Input: dimensioned drawing with shaded views. Units: mm. Origin: part minimum x, y, z. Give positions to 0.01 mm unless a question says otherwise; leave off trailing zeros. Order: outer loops, then holes, each group sorted by start corner. A loop starts at its lowest first (then second) coordinate and runs counter-clockwise, first axis right, second up. Notation, with made-up numbers: M -9,8.5 L 9,8.5 A17 cw 9,12.5 Z; hole C 21.25,10 d11. An arc over 180 degrees is marked long. Answer in a Markdown table with one row per item. Add a question column.
(1) Material intervals for line 1 along Y through (x, z) = (6.5, 1.75); line 2 along Y through (x, z) = (7, 0.3) (1 decimal); line 3 along X through (y, z) = (21, 0.25) (1 decimal), sorted ascending.
(2) Mould query, pull axis Y, two halves, no side actions, for the marked faces 1, 2 and 3. Classes: pulls with the +Y half, pulls with the -Y half, needs draft (parallel to the pull), parting line crosses it, or undercut.
(3) Section query D-D, the plane y = 2.25. Return loops of the section in (x, z) (1 decimal), plus the area to 3 significant figures.
(4) Pin query (flat end, axial travel): P1, Ø6, axis at x = 8.04, y = 19.05, coming from the +Z side (3 decimals); P2, Ø1.5, axis at y = 10, z = 1.5, coming from the -X side. Return the tip coordinate at first contact, or that it passes through.
(5) Section query C-C, the plane x = 15.25. Return loops of the section in (y, z) (1 decimal), plus the area to 3 significant figures.
(6) Section query A-A, the plane y = 19.05. Return loops of the section in (x, z) (1 decimal).
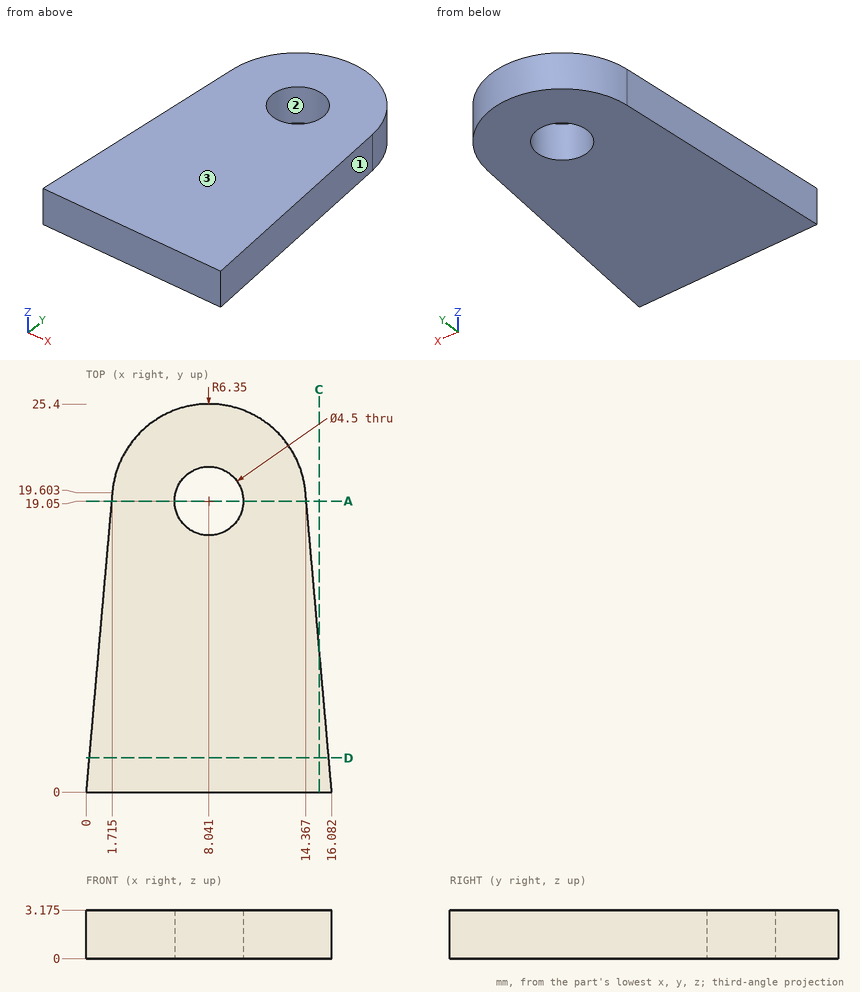
Values follow:
| question | item | result |
|---|---|---|
| 1 | line 1 | y = 0 to 17.41, 20.69 to 25.21 |
| 1 | line 2 | y = 0 to 17.1, 21 to 25.3 |
| 1 | line 3 | x = 2 to 6.9, 9.2 to 14.1 |
| 2 | face 1 | pulls with the +Y half |
| 2 | face 2 | undercut |
| 2 | face 3 | needs draft |
| 3 | outline | M 0.2,0 L 15.9,0 L 15.9,3.2 L 0.2,3.2 Z |
| 3 | area | 49.8 mm² |
| 4 | P1 | stops at z = 3.175 |
| 4 | P2 | stops at x = 0.81 |
| 5 | outline | M 0,0 L 9.5,0 L 9.5,3.2 L 0,3.2 Z |
| 5 | area | 30.2 mm² |
| 6 | outline | M 1.7,0 L 5.8,0 L 5.8,3.2 L 1.7,3.2 Z; M 10.3,0 L 14.4,0 L 14.4,3.2 L 10.3,3.2 Z |
